Read the model definition and answer for the solid it produces. Units are mm, in the model's axes. A direction names the side the tool comes from. Coordinates: 2 decimals unless noted, no trailing zeros. Order: outer loops, then holes, each group sorted by start corner. A loop starts at its lowest first (then second) coordinate and runs counter-clockwise, first axis right, second up. Notation, with made-up numbers: M 9.25,-10.5 L 28.25,-10.5 A8 cw 28.25,-1.5 Z; hole C 47.25,-5 d10. An arc over 180 degrees is marked long. One line per question, with ' | ' between items. Start each with the question number.
1) Find section A-A, the plane z = -16. Write down the section's boundary in (x, y).
2) Consider probe 1 along Z at (x, y) = (-20, 9.5); probe 2 along X at (y, z) = (7.5, 18); probe 3 along X at (y, z) = (7.75, 19.5). Determine where each line is inside the solid, lowest interval first.
3) Find section B-B, the plane y = 6.5. Write down the section's boundary in (x, z).
4) The mould has two halves that part along Z. Classify faces 3 (the face through (-22.5, 8, -20)), 4 (the face through (-26.07, 2.54, -43.5)), 5 (the face through (0, 0, -1)): +Z half, -Z half, draft (parallel to the pull), parting line (faces both ways), or undercut.
5) Given P1, Ø6, axis at x = -13, y = 6, coming from the -Z side; P2, Ø4, axis at x = -20.5, y = 7.5, coming from the +Z side; P3, Ø3, axis at y = 9, z = -12, coming from the -X side; P4, Ø2.5, axis at y = 7, z = 22.5, coming from the +X side, each flat-ended and moving along its own axis, determine where each tip first touches the part or whether it passes through.
6) A tool of negligible diameter and unlimited length cuts with its end or side. For faces 1 (the face through (0, 10, -1)), 2 (the face through (-22.5, 8, 20)), from which of +Z, -Z, +X, -X, +Y, -Y can it reach the whole face along a straight path? Write none if from no direction.
from build123d import *

# Parameters (mm, degrees)
SKETCH_2_W          = 55
SKETCH_2_H          = 90
EXTRUDE_1_DEPTH     = 10
FILLET_1_R          = 5
FILLET_2_R          = 5
FILLET_3_R          = 5
FILLET_4_R          = 5
SKETCH_3_W          = 5.5
SKETCH_3_H          = 10.5
CUT_EXTRUDE_1_DEPTH = 5


with BuildPart() as part:
    # 草图2 → 凸台-拉伸1 (new body)
    with BuildSketch(Plane(origin=(0, 0, 0), x_dir=(1, 0, 0), z_dir=(0, 1, 0))):
        Rectangle(SKETCH_2_W, SKETCH_2_H)
    extrude(amount=EXTRUDE_1_DEPTH)

    # 圆角1
    fillet_1_edges = [part.edges().sort_by_distance(p)[0] for p in [
        (-27.5, 10, 0),
    ]]
    fillet(fillet_1_edges, radius=FILLET_1_R)

    # 圆角2
    fillet_2_edges = [part.edges().sort_by_distance(p)[0] for p in [
        (-27.5, 2.5, -45),
        (-26.035533906, 8.535533906, -45),
        (2.5, 10, -45),
    ]]
    fillet(fillet_2_edges, radius=FILLET_2_R)

    # 圆角3
    fillet_3_edges = [part.edges().sort_by_distance(p)[0] for p in [
        (27.5, 2.5, -45),
        (27.5, 8.535533906, -43.535533906),
        (27.5, 10, 2.5),
    ]]
    fillet(fillet_3_edges, radius=FILLET_3_R)

    # 圆角4
    fillet_4_edges = [part.edges().sort_by_distance(p)[0] for p in [
        (0, 10, 45),
        (-27.5, 2.5, 45),
        (-26.035533906, 8.535533906, 45),
        (27.5, 2.5, 45),
        (26.035533906, 8.535533906, 45),
    ]]
    fillet(fillet_4_edges, radius=FILLET_4_R)

    # 草图3 → 切除-拉伸1 (cut)
    with BuildSketch(Plane(origin=(0, 10, 0), x_dir=(1, 0, 0), z_dir=(0, 1, 0))):
        with Locations((-19.75, 19.75)):
            Rectangle(SKETCH_3_W, SKETCH_3_H)
        with Locations((-19.75, -20.25)):
            Rectangle(SKETCH_3_W, SKETCH_3_H)
    extrude(amount=-CUT_EXTRUDE_1_DEPTH, mode=Mode.SUBTRACT)


solid = part.part
Report:
1) outline: M -27.5,0 L 27.5,0 L 27.5,5 A5 ccw 22.5,10 L -17,10 L -17,5 L -22.5,5 L -22.5,10 A5 ccw -27.5,5 Z
2) probe 1: z = -42.18 to -25, -14.5 to 15, 25.5 to 42.18 | probe 2: x = -26.83 to -22.5, -17 to 26.83 | probe 3: x = -26.68 to -22.5, -17 to 26.68
3) outline: M -27.27,-40 A4.77 ccw -22.5,-44.77 L 22.5,-44.77 A4.77 ccw 27.27,-40 L 27.27,40 A4.77 ccw 22.5,44.77 L -22.5,44.77 A4.77 ccw -27.27,40 Z; hole M -22.5,-25 L -17,-25 L -17,-14.5 L -22.5,-14.5 Z; hole M -22.5,15 L -17,15 L -17,25.5 L -22.5,25.5 Z
4) face 3: undercut | face 4: -Z half | face 5: draft
5) P1: stops at z = -45 | P2: stops at z = 44.97 | P3: stops at x = -26.83 | P4: stops at x = 27.44
6) face 1: +Z, -Z, +X, -X, +Y | face 2: +Y
